from build123d import *

# Parameters (mm, degrees)
CSK_FOR_0_FLAT_HEAD_MACHINE_SCREW_100_D           = 1.778
CSK_FOR_0_FLAT_HEAD_MACHINE_SCREW_100_CSINK_D     = 3.0226
CSK_FOR_0_FLAT_HEAD_MACHINE_SCREW_100_CSINK_ANGLE = 100
CIRPATTERN1_COUNT                                 = 12


with BuildPart() as part:
    # Sketch1 → Revolve1 (revolve)
    with BuildSketch(Plane.XY):
        with BuildLine():
            Line((-44.45, 0), (-38.1, 0))
            ThreePointArc((-38.1, 0), (-38.054138834, 0.213808772), (-37.924624138, 0.390000091))
            ThreePointArc((-37.924624138, 0.390000091), (-23.22414199, 9.855095754), (-6.35, 14.432818263))
            Line((-6.35, 14.432818263), (-6.35, 15.455036958))
            ThreePointArc((-6.35, 15.455036958), (-23.281489865, 10.940122909), (-38.1, 1.5875))
            Line((-38.1, 1.5875), (-44.45, 1.5875))
            Line((-44.45, 1.5875), (-44.45, 0))
        make_face()
    revolve(axis=Axis((0, 55, 0), (0, -1, 0)))

    # CSK for #0 Flat Head Machine Screw (100)1 (through all)
    with Locations(Plane(origin=(0, 1.5875, 0), x_dir=(1, 0, 0), z_dir=(0, 1, 0))):
        with Locations((-41.275, 0)):
            csk_for_0_flat_head_machine_screw_100 = CounterSinkHole(CSK_FOR_0_FLAT_HEAD_MACHINE_SCREW_100_D / 2, CSK_FOR_0_FLAT_HEAD_MACHINE_SCREW_100_CSINK_D / 2, counter_sink_angle=CSK_FOR_0_FLAT_HEAD_MACHINE_SCREW_100_CSINK_ANGLE)

    # CirPattern1: CSK for #0 Flat Head Machine Screw (100)1 ×12 about axis
    cirpattern1_axis = Axis((0, 0, 0), (0, 1, 0))
    for i in range(1, CIRPATTERN1_COUNT):
        add(csk_for_0_flat_head_machine_screw_100.rotate(cirpattern1_axis, i * 360 / CIRPATTERN1_COUNT), mode=Mode.SUBTRACT)


solid = part.part
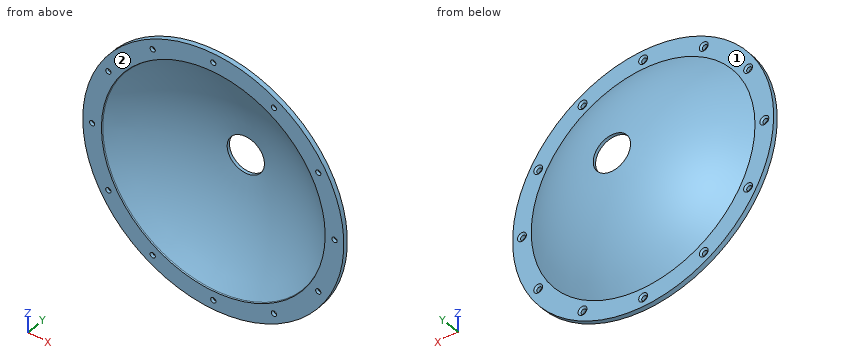
Can you work these out from the model? Positions are in its coordinate system, mm. Face numbers are marked on the shaded views. A direction names the side the tool comes from. Give positions to 0.01 mm unless a question says otherwise; leave off trailing zeros. Order: outer loops, then holes, each group sorted by start corner. A loop starts at its lowest first (then second) coordinate and runs counter-clockwise, first axis right, second up. Notation, with made-up numbers: M -24.75,47 L -4.75,47 A14 cw -4.75,65 Z; hole C 81,76 d3. An arc over 180 degrees is marked long. Use one line per item in the form item = value. Start each with the question number.
Item 1: For the marked faces 1 and 2, which set-ups out of +Z, -Z, +X, -X, +Y, -Y let a thin tool reach every point of the face, with its end or its side?
Item 2: Will these pins go through, and if not, where does the flat tip stop? pin 1 Ø6 at (x, z) = (28, -26.5) entering from +Y; pin 2 Ø2 at (x, z) = (-35.75, -20.64) entering from +Y; pin 3 Ø4 at (y, z) = (6.5, 10.5) entering from +X.
Item 3: If I drill on line 1 along Y through (x, z) = (4, -40.5); line 2 along X through (y, z) = (3.5, 10.5); line 3 along Z through (x, y) = (-5.5, 4), over which ranges is the centre line in solid material (lowest first)?
Item 4: If we section it at A-A (y = 3): Write out the boundary of the cut face in (x, z).
Outcome:
q1.face_1 = +Y
q1.face_2 = +Z, -Z, +X, -X, -Y
q2.pin_1 = 3.67
q2.pin_2 = 1.16
q2.pin_3 = 32.88
q3.line_1 = 0 to 1.59
q3.line_2 = -34.2 to -32.44, 32.44 to 34.2
q3.line_3 = -34.69 to -32.96, 32.96 to 34.69
q4.outline = C 0,0 d72.81; hole C 0,0 d69.52
